from build123d import *

# Parameters (mm, degrees)
F0_W         = 20
F0_H         = 45
F0_R         = 4
F0_R_2       = 6.15
F1_DEPTH     = 4
F1_FACE_W    = 20
F1_FACE_H    = 45
F1_FACE_R    = 4
F1_FACE_R_2  = 6.15
F0_R_3       = 2
F0_R_4       = 2.75
F2_DEPTH     = 0.5
F4_T1_DEPTH  = 97.9025398997
F5_DEPTH     = 5
F3_W         = 20
F3_H         = 10
F6_DEPTH     = 6
F7_R         = 3.2
F8_DEPTH     = 25
F10_R        = 9.99999
F11_R        = 1
F12_DEPTH    = 25
F13_T1_DEPTH = 45


# Not quite as in the source:
# - a fillet or chamfer that OpenCascade refuses, or shapes differently, is made with other operations: its cross-section is extruded or revolved along the edge and cut away or added
# - a fillet or chamfer is up to 0.001 mm smaller than in the source, because OpenCascade refuses the exact size
# - a feature of the source that left no trace in its solid (it failed there, or was rolled back) is left out


with BuildPart() as f1:
    # F0 (on Top) → F1 (new body)
    with BuildSketch(Plane.XY):
        with Locations((10, 22.5)):
            Rectangle(F0_W, F0_H)
        with Locations((10, 10)):
            Circle(F0_R, mode=Mode.SUBTRACT)
        with Locations((10, 35)):
            Circle(F0_R_2, mode=Mode.SUBTRACT)
    extrude(amount=F1_DEPTH)

    # F1_face (on face) + F0 (on Top) → F2 (join)
    with BuildSketch(Plane(origin=(10, 21.3275360022, 4), x_dir=(1, 0, 0), z_dir=(0, 0, 1))):
        with Locations((0, 1.1724639978)):
            Rectangle(F1_FACE_W, F1_FACE_H)
        with Locations((0, -11.3275360022)):
            Circle(F1_FACE_R, mode=Mode.SUBTRACT)
        with Locations((0, 13.6724639978)):
            Circle(F1_FACE_R_2, mode=Mode.SUBTRACT)
    with BuildSketch(Plane.XY):
        with Locations((10, 35)):
            Circle(F0_R_2)
        with Locations((10, 35)):
            Circle(F0_R_3, mode=Mode.SUBTRACT)
        with Locations((10, 10)):
            Circle(F0_R_4)
    extrude(amount=F2_DEPTH)

    # F4: chamfer of 15 x 4 on 2 edges, made by hand

    # F4_s2 → F4_t1 (cut)
    with BuildSketch(Plane.YZ.offset(-38.9512699498)):
        Polygon((0, 0.5), (15, 4.5), (0, 4.5), align=None)
        Polygon((30, 4.5), (45, 0.5), (45, 4.5), align=None)
    extrude(amount=F4_T1_DEPTH, mode=Mode.SUBTRACT)

    # F0 (on Top) → F5 (join)
    with BuildSketch(Plane.XY):
        with Locations((10, 10)):
            Circle(F0_R)
        with Locations((10, 10)):
            Circle(F0_R_4, mode=Mode.SUBTRACT)
    extrude(amount=F5_DEPTH)

    # F3 (on face) → F6 (join)
    with BuildSketch(Plane.XY.offset(4.5)):
        with Locations((10, 20)):
            Rectangle(F3_W, F3_H)
    extrude(amount=F6_DEPTH)

    # F7 (on face) → F8 (cut)
    with BuildSketch(Plane(origin=(0, 0, 0), x_dir=(0, -1, 0), z_dir=(-1, 0, 0))):
        with Locations((-20, 6)):
            Circle(F7_R)
    extrude(amount=-F8_DEPTH, mode=Mode.SUBTRACT)

    # F10 (radius 10 in the source; OpenCascade refuses exactly that, so slightly less here)
    f10_edges = [f1.edges().sort_by_distance(p)[0] for p in [
        (0, 45, 0.25),
        (20, 45, 0.25),
    ]]
    fillet(f10_edges, radius=F10_R)

    # F11 (on face) → F12 (cut)
    with BuildSketch(Plane.XY.offset(10.5)):
        with Locations((4, 20)):
            Circle(F11_R)
        with Locations((16, 20)):
            Circle(F11_R)
    extrude(amount=-F12_DEPTH, mode=Mode.SUBTRACT)

    # F13: fillet of radius 5 on 2 edges, made by hand

    # F13_s2 → F13_t1 (cut)
    with BuildSketch(Plane.YZ.offset(-12.5)):
        with BuildLine():
            ThreePointArc((25, 5.5), (23.5355339059, 9.0355339059), (20, 10.5))
            Line((20, 10.5), (25, 10.5))
            Line((25, 10.5), (25, 5.5))
        make_face()
        with BuildLine():
            ThreePointArc((20, 10.5), (16.4644660941, 9.0355339059), (15, 5.5))
            Line((15, 5.5), (15, 10.5))
            Line((15, 10.5), (20, 10.5))
        make_face()
    extrude(amount=F13_T1_DEPTH, mode=Mode.SUBTRACT)


solid = f1.part
Can you work these out from the model? Positions are in its coordinate system, mm. A direction names the side the tool comes from. Give positions to 0.01 mm unless a question says otherwise; leave off trailing zeros. Write each loop counter-clockwise with the first axis right and the second up, starting at its lowest first coordinate (ties: lowest second). Pieces come first, ordered by that corner, then holes. Notation, with made-up numbers: (-2.5, 50) -> (20.5, 50) arc R25 ccw to (20.5, 80) -> close; hole circle Ø7 at (-28.75, -19). An arc over 180 degrees is marked (long way). Answer as a JSON object with one key per item and string values. Group by question number.
Item 1: Suppose I cut it at C-C (x = 18.5). Please give me the cut outline in (y, z).
Item 2: We'd pull the mould along X, two halves only. Please class faces 4 (the face through (10, 15, 5)), 5 (the face through (20, 21.1, 2.8)), 6 (the face through (15.263, 20.676, 9.78)), 7 (the face through (0, 21.1, 2.8)): +X half, -X half, draft (parallel to the pull), parting line (faces both ways), or undercut.
Item 3: Please list where these lines run through material, in increasing order: line 1 (X direction, y = 20, z = 9.4); line 2 (Y direction, x = 10, z = 2.6); line 3 (Y direction, x = 10, z = 3.65). Write a range as [from, to].
Item 4: Suppose I cut it at B-B (y = 10). Please give me the cut outline in (x, z).
Item 5: For faces 1 (the face through (16, 19, 2)), 2 (the face through (10, 28, 4.5)), 3 (the face through (8.667, 28.996, 2.028)), which set-ups out of +Z, -Z, +X, -X, +Y, -Y let a thin tool reach every point of the face, with its end or its side?
Item 6: I'm going to push flat-ended pins straight in: P1, Ø1.2, axis at x = 4, y = 20, coming from the -Z side; P2, Ø1.6, axis at x = 10, y = 10, coming from the +Z side; P3, Ø0.8, axis at x = 7, z = 5, coming from the -Y side; P4, Ø5.5, axis at x = 13.5, y = 27, coming from the +Z side. Where does each tip first touch, or does it pass through?
Item 7: Suppose I cut it at D-D (x = 2.25). Please give me the cut outline in (y, z).
Item 8: Suppose I cut it at A-A (z = 6). Please give me the cut outline in (x, y).
Findings:
{
 "1": {"outline": "(0, 0) -> (40.27, 0) -> (40.27, 1.76) -> (30, 4.5) -> (25, 4.5) -> (25, 5.5) arc R5 ccw to (15, 5.5) -> (15, 4.5) -> (0, 0.5) -> close; hole circle Ø6.4 at (20, 6)"},
 "2": {"face 4": "draft", "face 5": "+X half", "face 6": "undercut", "face 7": "-X half"},
 "3": {"line 1": "x = [0, 3], [5, 15], [17, 20]", "line 2": "y = [6, 7.25], [12.75, 28.85]", "line 3": "y = [6, 7.25], [12.75, 17.83], [22.17, 28.85]"},
 "4": {"outline": "(0, 0) -> (20, 0) -> (20, 3.17) -> (14, 3.17) -> (14, 5) -> (12.75, 5) -> (12.75, 0.5) -> (7.25, 0.5) -> (7.25, 5) -> (6, 5) -> (6, 3.17) -> (0, 3.17) -> close"},
 "5": {"face 1": "+Z, -Z", "face 2": "+Z, +X, -X, +Y", "face 3": "+Z"},
 "6": {"P1": "passes through", "P2": "stops at z = 0.5", "P3": "stops at y = 6.96", "P4": "stops at z = 8.13"},
 "7": {"outline": "(0, 0) -> (41.32, 0) -> (41.32, 1.48) -> (30, 4.5) -> (25, 4.5) -> (25, 5.5) arc R5 ccw to (15, 5.5) -> (15, 4.5) -> (0, 0.5) -> close; hole circle Ø6.4 at (20, 6)"},
 "8": {"outline": "(0, 15.03) -> (20, 15.03) -> (20, 16.8) -> (0, 16.8) -> close; (0, 23.2) -> (20, 23.2) -> (20, 24.97) -> (0, 24.97) -> close"}
}
